```python
from build123d import *

# Parameters (mm, degrees)
F0_W     = 500
F0_H     = 464
F1_DEPTH = 9.5


with BuildPart() as f1:
    # F0 (on Top) → F1 (new body)
    with BuildSketch(Plane.XY):
        with Locations((199.084524, 215.949913)):
            Rectangle(F0_W, F0_H)
        Polygon((30.084524, 312.385261), (199.084524, 312.385261), (368.084524, 312.385261), (368.084524, 42.385261), (30.084524, 42.385261), align=None, mode=Mode.SUBTRACT)
    extrude(amount=F1_DEPTH)


solid = f1.part
```
Design review of the part built by this model. Coordinates are the model's own, in mm. Coordinates: 2 decimals unless noted, no trailing zeros. Write each loop counter-clockwise with the first axis right and the second up, starting at its lowest first coordinate (ties: lowest second). Pieces come first, ordered by that corner, then holes.
1) To check wall thickness, follow L1, parallel to Y at x = 114.5, z = 6.5; L2, parallel to X at y = 96, z = 2. State the ranges of each line that lie inside material, in increasing order.
2) Add section C-C (z = 3). Write out the cut boundary in (x, y).
3) Add section B-B (y = 121.5). Write out the cut boundary in (x, z).
4) Add section A-A (x = 157.5). Write out the cut boundary in (y, z).
5) Insertion check: pin 1 (2 mm diameter, centred on x = 149.5, y = 399.5, fed in from -Z). The pin has a flat end and moves straight along its axis. Give the tip position at first contact, or say it passes through.
Check result:
1. L1: y = -16.05 to 42.39, 312.39 to 447.95
1. L2: x = -50.92 to 30.08, 368.08 to 449.08
2. outline: (-50.92, -16.05) - (449.08, -16.05) - (449.08, 447.95) - (-50.92, 447.95) - close; hole (30.08, 42.39) - (368.08, 42.39) - (368.08, 312.39) - (30.08, 312.39) - close
3. outline: (-50.92, 0) - (30.08, 0) - (30.08, 9.5) - (-50.92, 9.5) - close; (368.08, 0) - (449.08, 0) - (449.08, 9.5) - (368.08, 9.5) - close
4. outline: (-16.05, 0) - (42.39, 0) - (42.39, 9.5) - (-16.05, 9.5) - close; (312.39, 0) - (447.95, 0) - (447.95, 9.5) - (312.39, 9.5) - close
5. pin 1: stops at z = 0
